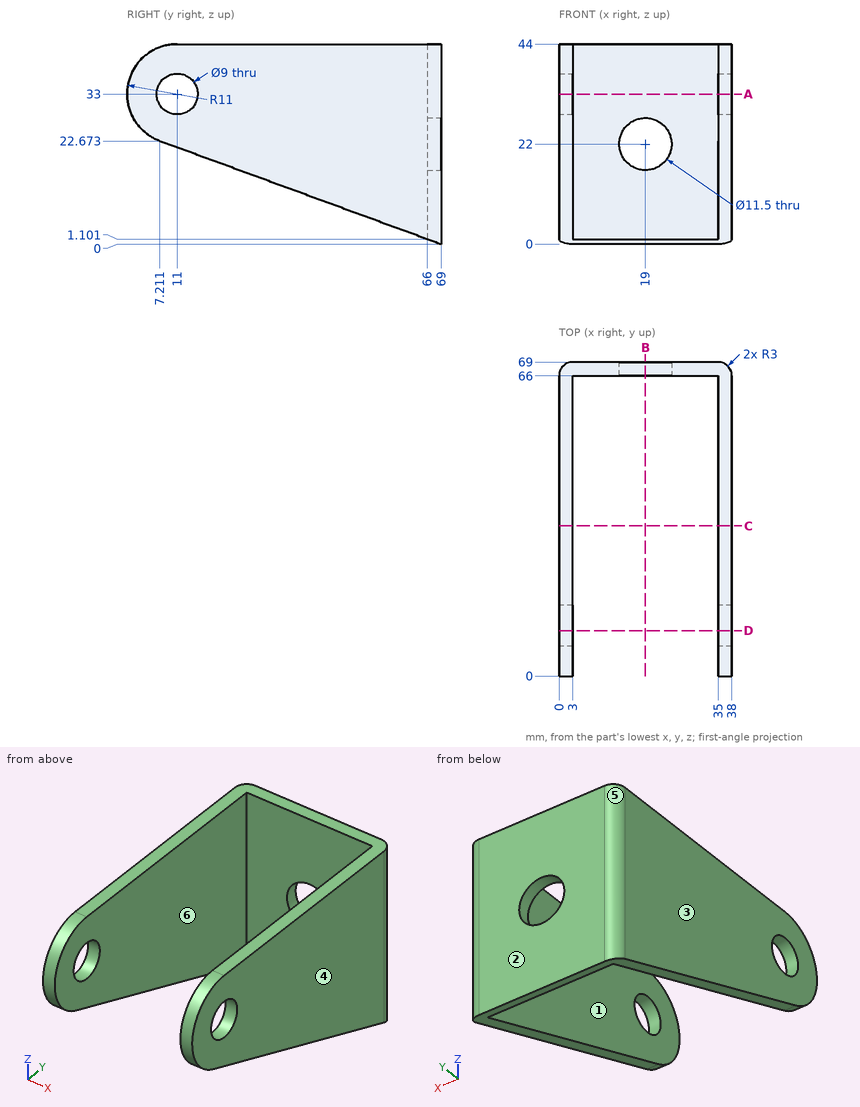
Geometry check sheet. Reference: drawing and pictorial views, mm from the part's lowest x, y, z. A direction names the side the tool comes from. Give positions to 0.01 mm unless a question says otherwise; leave off trailing zeros. Order: outer loops, then holes, each group sorted by start corner. A loop starts at its lowest first (then second) coordinate and runs counter-clockwise, first axis right, second up. Notation, with made-up numbers: (70.5, 88.25) - (118.5, 88.25) arc R32 ccw to (118.5, 126.25) - close; hole circle Ø3 at (39, 1). An arc over 180 degrees is marked (long way). Answer as CSV lines item,"result". Start each with the question number.
Item 1: Mould release check, pull along X, two halves, no side actions. Record for the marked faces 1, 2, 3 and 4: released by +X, released by -X, zero draft, split by the parting line, or undercut.
Item 2: Access from +Z, -Z, +X, -X, +Y, -Y to the whole of each face (thin tool, end or side, straight path). Record for the marked faces 5 and 6.
Item 3: Section check D-D, the plane y = 10. State how many separate pieces and enclosed holes the cut face has.
Item 4: Section check C-C, the plane y = 33. Record the boundary of the cut face in (x, z).
Item 5: Gauge pin test, flat ends, axial feed: pin 1 (2 mm diameter, centred on y = 14, z = 18.5, fed in from +X); pin 2 (8 mm diameter, centred on x = 24, z = 24.5, fed in from -Y). Record the tip position at first contact, or that the pin passes through.
Item 6: Section check B-B, the plane x = 19. Record the boundary of the cut face in (y, z).
Item 7: Section check A-A, the plane z = 33. Record the boundary of the cut face in (x, y).
Item 8: Material ranges on L1, parallel to X at y = 23, z = 27; L2, parallel to Y at x = 15, z = 15; L3, parallel to X at y = 66.85, z = 22, recorded low to high.
Filled in:
1,face 1,"undercut"
1,face 2,"zero draft"
1,face 3,"released by -X"
1,face 4,"released by +X"
2,face 5,"+Z, -Z, -X, +Y"
2,face 6,"+Z, -Z, -Y"
3,separate pieces,"4"
3,enclosed holes,"0"
4,outline,"(0, 13.21) - (3, 13.21) - (3, 44) - (0, 44) - close; (35, 13.21) - (38, 13.21) - (38, 44) - (35, 44) - close"
5,pin 1,"through"
5,pin 2,"y = 66"
6,outline,"(66, 1.1) - (69, 0) - (69, 16.25) - (66, 16.25) - close; (66, 27.75) - (69, 27.75) - (69, 44) - (66, 44) - close"
7,outline,"(0, 0) - (3, 0) - (3, 6.5) - (0, 6.5) - close; (0, 15.5) - (3, 15.5) - (3, 66) - (35, 66) - (35, 15.5) - (38, 15.5) - (38, 66) arc R3 ccw to (35, 69) - (3, 69) arc R3 ccw to (0, 66) - close; (35, 0) - (38, 0) - (38, 6.5) - (35, 6.5) - close"
8,L1,"0 to 3, 35 to 38"
8,L2,"66 to 69"
8,L3,"0.12 to 13.25, 24.75 to 37.88"
